Verification items for the finished model (mm, model axes). Give positions to 0.01 mm unless a question says otherwise; leave off trailing zeros. Write each loop counter-clockwise with the first axis right and the second up, starting at its lowest first coordinate (ties: lowest second). Pieces come first, ordered by that corner, then holes. Notation, with made-up numbers: M 23,79 L 73,79 A20 ccw 73,118 Z; hole C 36.25,5 d8. An arc over 180 degrees is marked long. Write item = value, one per line.
from build123d import *

# Parameters (mm, degrees)
ESQUISSE1_R        = 4
BOSS_EXTRU_1_DEPTH = 13


with BuildPart() as part:
    # Esquisse1 → Boss.-Extru.1 (new body)
    with BuildSketch(Plane.XY):
        with BuildLine():
            Line((-34, -8), (34, -8))
            ThreePointArc((34, -8), (38.242640687, -6.242640687), (40, -2))
            Line((40, -2), (40, 2))
            ThreePointArc((40, 2), (38.242640687, 6.242640687), (34, 8))
            Line((34, 8), (-34, 8))
            ThreePointArc((-34, 8), (-38.242640687, 6.242640687), (-40, 2))
            Line((-40, 2), (-40, -2))
            ThreePointArc((-40, -2), (-38.242640687, -6.242640687), (-34, -8))
        make_face()
        with Locations(Location((-32, 0, 0), (0, 0, 180))):
            Circle(ESQUISSE1_R, mode=Mode.SUBTRACT)
        with Locations(Location((32, 0, 0), (0, 0, 180))):
            Circle(ESQUISSE1_R, mode=Mode.SUBTRACT)
    extrude(amount=BOSS_EXTRU_1_DEPTH)


solid = part.part
1) Cross-section at A-A on y = 0. Record the boundary of the cut face in (x, z).
From the geometry:
outline = M -40,0 L -36,0 L -36,13 L -40,13 Z; M -28,0 L 28,0 L 28,13 L -28,13 Z; M 36,0 L 40,0 L 40,13 L 36,13 Z
2) Material ranges on probe 1 along Y at (x, z) = (32, 9); probe 2 along X at (y, z) = (-0.5, 9); probe 3 along X at (y, z) = (3.5, 10.75), recorded low to high. Write a range as from..to.
From the geometry:
probe_1 = -8..-4, 4..8
probe_2 = -40..-35.97, -28.03..28.03, 35.97..40
probe_3 = -39.81..-33.94, -30.06..30.06, 33.94..39.81
3) Cross-section at D-D on y = -6.5. Record the boundary of the cut face in (x, z), plus the area to 3 significant figures.
From the geometry:
outline = M -37.97,0 L 37.97,0 L 37.97,13 L -37.97,13 Z
area = 987 mm^2
4) Cross-section at C-C on x = -32. Record the boundary of the cut face in (y, z), plus the area to 3 significant figures.
From the geometry:
outline = M -8,0 L -4,0 L -4,13 L -8,13 Z; M 4,0 L 8,0 L 8,13 L 4,13 Z
area = 104 mm^2
5) Cross-section at B-B on z = 5. Record the boundary of the cut face in (x, y).
From the geometry:
outline = M -40,-2 A6 ccw -34,-8 L 34,-8 A6 ccw 40,-2 L 40,2 A6 ccw 34,8 L -34,8 A6 ccw -40,2 Z; hole C -32,0 d8; hole C 32,0 d8
6) Draft check along X on faces 1 (the cylindrical face through (-28.8, 2.4, 6.4)), 2 (the flat face through (0, -8, 6)), 3 (the cylindrical face through (-38.196, 6.289, 6.409)). Enter one of: +X half, -X half, draft (parallel to the pull), parting line (faces both ways), or undercut.
From the geometry:
face_1 = undercut
face_2 = draft
face_3 = -X half
